Geometry: final body of the model. Coordinates: model frame, mm. Face numbers are marked on the shaded views. Round coordinates to 2 decimals unless told otherwise and drop trailing zeros. Loops run counter-clockwise (first coordinate to the right, second up) from the corner with the lowest first, then second, coordinate; pieces in that order, holes last. Notation, with made-up numbers: (19, 2) -> (51, 2) arc R32 cw to (51, 38) -> close; hole circle Ø3 at (84, -16). An arc over 180 degrees is marked (long way). Answer in a Markdown table with one row per item.
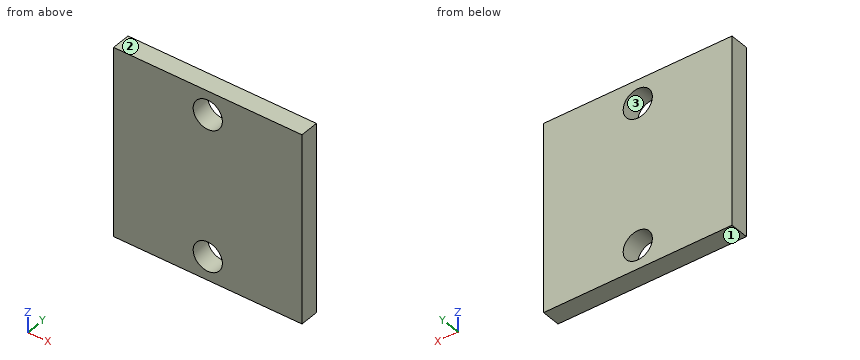
Autodesk Inventor part; units mm, degrees
ref_plane "YZ Plane" through (0, 0, 0) normal (1, 0, 0) x (0, 1, 0)
ref_plane "XZ Plane" through (0, 0, 0) normal (0, 1, 0) x (-1, 0, 0)
ref_plane "XY Plane" through (0, 0, 0) normal (0, 0, 1) x (1, 0, 0)
sketch "Sketch1" plane through (0, 0, 0) normal (0, 1, 0) x (-1, 0, 0)
  line L0 (0, 0) -> (-100, 0)
  line L1 (-100, 0) -> (-100, -100)
  line L2 (-100, -100) -> (0, -100)
  line L3 (0, -100) -> (0, 0)
  dimension "d0" = 100
  dimension "d1" = 100
extrude "Extrusion1" add sketch "Sketch1" along normal blind 10
sketch "Sketch2" plane through (0, 10, 0) normal (0, 1, 0) x (1, 0, 0)
  circle A0 centre (50, 12.5) radius 7.75
  circle A1 centre (50, 87.5) radius 7.75
  line L0 (0, 0) -> (100, 0)
  line L1 (0, 100) -> (0, 0)
  line L2 (100, 100) -> (0, 100)
  dimension "d4" = 15.5
  dimension "d5" = 15.5
  dimension "d6" = 12.5
  dimension "d7" = 50
  dimension "d8" = 12.5
  dimension "d9" = 50
extrude "Extrusion2" cut sketch "Sketch2" against normal blind 10
properties part number "Ba" material "Wood (Oak)"
Item 1: Cut plane B-B (x = 50). Output: boundary loops of the cut face in (y, z).
Answer:
| item | result |
|---|---|
| outline | (0, -100) -> (10, -100) -> (10, -95.25) -> (0, -95.25) -> close; (0, -79.75) -> (10, -79.75) -> (10, -20.25) -> (0, -20.25) -> close; (0, -4.75) -> (10, -4.75) -> (10, 0) -> (0, 0) -> close |
Item 2: Cut plane C-C (y = 8). Output: boundary loops of the cut face in (x, z).
Answer:
| item | result |
|---|---|
| outline | (0, -100) -> (100, -100) -> (100, 0) -> (0, 0) -> close; hole circle Ø15.5 at (50, -87.5); hole circle Ø15.5 at (50, -12.5) |
Item 3: Cut plane A-A (z = -12.5). Output: boundary loops of the cut face in (x, y), then the cut area to 3 significant figures.
Answer:
| item | result |
|---|---|
| outline | (0, 0) -> (42.25, 0) -> (42.25, 10) -> (0, 10) -> close; (57.75, 0) -> (100, 0) -> (100, 10) -> (57.75, 10) -> close |
| area | 845 mm² |
Item 4: Draft query along Z for the marked faces 1, 2 and 3. Return one class per face: pulls with the +Z half, pulls with the -Z half, needs draft (parallel to the pull), parting line crosses it, or undercut.
Answer:
| item | result |
|---|---|
| face 1 | pulls with the -Z half |
| face 2 | pulls with the +Z half |
| face 3 | undercut |
Item 5: Cut plane D-D (z = -86). Output: boundary loops of the cut face in (x, y).
Answer:
| item | result |
|---|---|
| outline | (0, 0) -> (42.4, 0) -> (42.4, 10) -> (0, 10) -> close; (57.6, 0) -> (100, 0) -> (100, 10) -> (57.6, 10) -> close |
Item 6: Line query: probe 1 along Z at (x, y) = (50, 2.5); probe 2 along X at (y, z) = (5.5, -12.5); probe 3 along Z at (x, y) = (57, 9.75). Output: solid intervals per line, ascending. Write a range as [from, to].
Answer:
| item | result |
|---|---|
| probe 1 | z = [-100, -95.25], [-79.75, -20.25], [-4.75, 0] |
| probe 2 | x = [0, 42.25], [57.75, 100] |
| probe 3 | z = [-100, -90.83], [-84.17, -15.83], [-9.17, 0] |
